The figure shows three views and two pictorial views of one solid part (mm, origin at its lowest corner). Answer the questions. A direction names the side the tool comes from. Round coordinates to 2 decimals unless told otherwise and drop trailing zeros. Write each loop counter-clockwise with the first axis right and the second up, starting at its lowest first coordinate (ties: lowest second). Pieces come first, ordered by that corner, then holes.
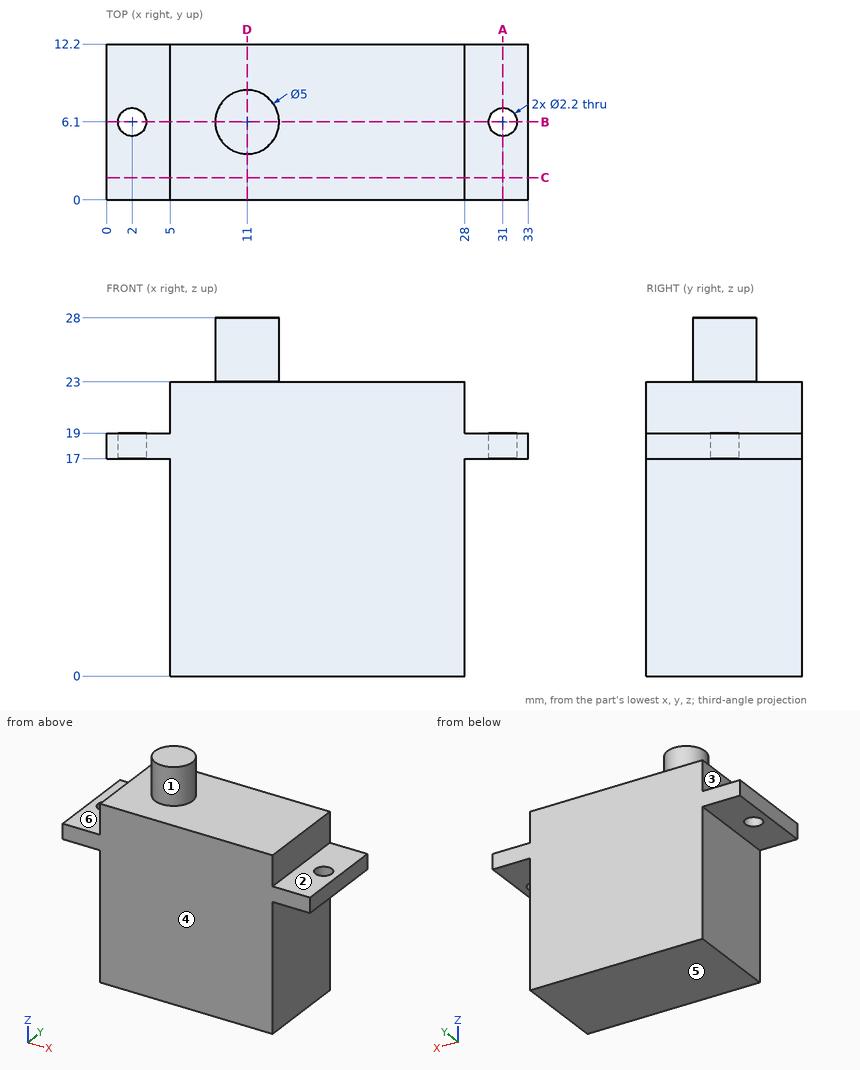
Q1. Section C-C (y = 1.75) is taken. Determine the outline of the cut face in (x, z).
Verdict:
outline: (0, 17) - (5, 17) - (5, 0) - (28, 0) - (28, 17) - (33, 17) - (33, 19) - (28, 19) - (28, 23) - (5, 23) - (5, 19) - (0, 19) - close
Q2. Determine the mould class of the marked faces 4, 5 and 6 for opening direction Z: pulls with the +Z half, pulls with the -Z half, needs draft (parallel to the pull), parting line crosses it, or undercut.
Verdict:
face 4: needs draft
face 5: pulls with the -Z half
face 6: pulls with the +Z half
Q3. Section B-B (y = 6.1) is taken. Determine the outline of the cut face in (x, z), then the cut area to 3 significant figures.
Verdict:
outline: (0, 17) - (0.9, 17) - (0.9, 19) - (0, 19) - close; (3.1, 17) - (5, 17) - (5, 0) - (28, 0) - (28, 17) - (29.9, 17) - (29.9, 19) - (28, 19) - (28, 23) - (13.5, 23) - (13.5, 28) - (8.5, 28) - (8.5, 23) - (5, 23) - (5, 19) - (3.1, 19) - close; (32.1, 17) - (33, 17) - (33, 19) - (32.1, 19) - close
area: 565 mm2
Q4. Which of the six approach directions +Z, -Z, +X, -X, +Y, -Y give full straight-line access (tool end or side, diameter ignored) to the marked faces 1, 2 and 3?
Verdict:
face 1: +Z
face 2: +Z, +X, +Y, -Y
face 3: +Z, -X, +Y, -Y
Q5. Flat-ended cylindrical pins translate along their axes: pin 1 Ø1.5 at (y, z) = (4.5, 3.5) entering from -X; pin 2 Ø1 at (y, z) = (11, 9) entering from +X; pin 3 Ø2.5 at (x, y) = (1.5, 8.5) entering from +Z; pin 4 Ø2 at (x, y) = (2, 6.1) entering from -Z. Find the tip coordinate at first contact, or state that the pin passes through.
Verdict:
pin 1: stops at x = 5
pin 2: stops at x = 28
pin 3: stops at z = 19
pin 4: passes through
Q6. Section A-A (x = 31) is taken. Determine the outline of the cut face in (y, z).
Verdict:
outline: (0, 17) - (5, 17) - (5, 19) - (0, 19) - close; (7.2, 17) - (12.2, 17) - (12.2, 19) - (7.2, 19) - close
Q7. Straight lines are drawn through the part: probe 1 along Y at (x, z) = (2, 18); probe 2 along Z at (x, y) = (6, 3.5); probe 3 along Z at (x, y) = (31, 0.75). For each, find the intervals that lie inside material, in ascending order.
Verdict:
probe 1: y = 0 to 5, 7.2 to 12.2
probe 2: z = 0 to 23
probe 3: z = 17 to 19
Q8. Section D-D (x = 11) is taken. Determine the outline of the cut face in (y, z), then the cut area to 3 significant figures.
Verdict:
outline: (0, 0) - (12.2, 0) - (12.2, 23) - (8.6, 23) - (8.6, 28) - (3.6, 28) - (3.6, 23) - (0, 23) - close
area: 306 mm2
